from build123d import *

# Parameters (mm, degrees)
SKETCH_1_R           = 155
EXTRUDE_1_DEPTH      = 5
SKETCH_16_R          = 1.5
CUT_EXTRUDE_15_DEPTH = 220.260119493
SKETCH_17_R          = 1.5
SKETCH_17_R_2        = 20.5
CUT_EXTRUDE_16_DEPTH = 220.260119493
SKETCH_19_R          = 2
SKETCH_19_R_2        = 1.5
CUT_EXTRUDE_17_DEPTH = 220.260119493
CUT_EXTRUDE_18_DEPTH = 220.260119493
SKETCH_21_R          = 1.5
CUT_EXTRUDE_19_DEPTH = 220.260119493
SKETCH_22_R          = 1.5
SKETCH_22_W          = 78
SKETCH_22_H          = 51
CUT_EXTRUDE_20_DEPTH = 220.260119493


with BuildPart() as part:
    # 草图1 → 凸台-拉伸1 (new body)
    with BuildSketch(Plane.XY):
        Circle(SKETCH_1_R)
    extrude(amount=EXTRUDE_1_DEPTH)

    # 草图16 → 切除-拉伸15 (cut, through all)
    with BuildSketch(Plane.XY.offset(5)):
        with Locations((0, 148)):
            Circle(SKETCH_16_R)
        with Locations((104.651803616, 104.651803616)):
            Circle(SKETCH_16_R)
        with Locations((148, 0)):
            Circle(SKETCH_16_R)
        with Locations((104.651803616, -104.651803616)):
            Circle(SKETCH_16_R)
        with Locations((0, -148)):
            Circle(SKETCH_16_R)
        with Locations((-104.651803616, -104.651803616)):
            Circle(SKETCH_16_R)
        with Locations((-148, 0)):
            Circle(SKETCH_16_R)
        with Locations((-104.651803616, 104.651803616)):
            Circle(SKETCH_16_R)
    extrude(amount=-CUT_EXTRUDE_15_DEPTH, mode=Mode.SUBTRACT)

    # 草图17 → 切除-拉伸16 (cut, through all)
    with BuildSketch(Plane.XY.offset(5)):
        with Locations((-80, -75)):
            Circle(SKETCH_17_R)
        with Locations((-80, -125)):
            Circle(SKETCH_17_R)
        with Locations((-80, -100)):
            Circle(SKETCH_17_R_2)
    extrude(amount=-CUT_EXTRUDE_16_DEPTH, mode=Mode.SUBTRACT)

    # 草图19 → 切除-拉伸17 (cut, through all)
    with BuildSketch(Plane.XY.offset(5)):
        with Locations((51.7, -68.3)):
            Circle(SKETCH_19_R)
        with Locations((43.2, -120.3)):
            Circle(SKETCH_19_R)
        with Locations((-43.2, -120.3)):
            Circle(SKETCH_19_R)
        with Locations((-51.7, -68.3)):
            Circle(SKETCH_19_R)
        with Locations((25.1, -72.7)):
            Circle(SKETCH_19_R_2)
        with Locations(Location((25.1, -122.7, 0), (0, 0, 180))):
            Circle(SKETCH_19_R_2)
        with Locations((-24.9, -122.7)):
            Circle(SKETCH_19_R_2)
        with Locations(Location((-24.9, -72.7, 0), (0, 0, 180))):
            Circle(SKETCH_19_R_2)
    extrude(amount=-CUT_EXTRUDE_17_DEPTH, mode=Mode.SUBTRACT)

    # 草图20 → 切除-拉伸18 (cut, through all)
    with BuildSketch(Plane.XY.offset(5)):
        with BuildLine():
            Line((-75, 42), (75, 42))
            ThreePointArc((75, 42), (82.071067812, 39.071067812), (85, 32))
            Line((85, 32), (85, -50))
            ThreePointArc((85, -50), (82.071067812, -57.071067812), (75, -60))
            Line((75, -60), (-75, -60))
            ThreePointArc((-75, -60), (-82.071067812, -57.071067812), (-85, -50))
            Line((-85, -50), (-85, 32))
            ThreePointArc((-85, 32), (-82.071067812, 39.071067812), (-75, 42))
        make_face()
    extrude(amount=-CUT_EXTRUDE_18_DEPTH, mode=Mode.SUBTRACT)

    # 草图21 → 切除-拉伸19 (cut, through all)
    with BuildSketch(Plane.XY.offset(5)):
        with Locations((95, 16)):
            Circle(SKETCH_21_R)
        with Locations((120, 16)):
            Circle(SKETCH_21_R)
        with Locations(Location((120, -34, 0), (0, 0, 180))):
            Circle(SKETCH_21_R)
        with Locations(Location((95, -34, 0), (0, 0, 180))):
            Circle(SKETCH_21_R)
        with Locations((-120, -34)):
            Circle(SKETCH_21_R)
        with Locations((-95, -34)):
            Circle(SKETCH_21_R)
        with Locations(Location((-120, 16, 0), (0, 0, 180))):
            Circle(SKETCH_21_R)
        with Locations(Location((-95, 16, 0), (0, 0, 180))):
            Circle(SKETCH_21_R)
    extrude(amount=-CUT_EXTRUDE_19_DEPTH, mode=Mode.SUBTRACT)

    # 草图22 → 切除-拉伸20 (cut, through all)
    with BuildSketch(Plane.XY.offset(5)):
        with Locations((-44, 129.5)):
            Circle(SKETCH_22_R)
        with Locations((44, 129.5)):
            Circle(SKETCH_22_R)
        with Locations((44, 70.5)):
            Circle(SKETCH_22_R)
        with Locations((-44, 70.5)):
            Circle(SKETCH_22_R)
        with Locations((0, 100)):
            Rectangle(SKETCH_22_W, SKETCH_22_H)
    extrude(amount=-CUT_EXTRUDE_20_DEPTH, mode=Mode.SUBTRACT)


solid = part.part
Build history of the part. All positions in model axes, mm. A direction names the side the tool comes from. Coordinates: 2 decimals unless noted, no trailing zeros. Order: outer loops, then holes, each group sorted by start corner. A loop starts at its lowest first (then second) coordinate and runs counter-clockwise, first axis right, second up. Notation, with made-up numbers: M 30.25,89 L 64.25,89 A15 cw 64.25,109 Z; hole C -20,58 d3. An arc over 180 degrees is marked long. One line per question, with ' | ' between items. Start each with the question number.
Q1. Saw through at D-D (y = 49). List the corners of the cut face in (x, z), then the cut area to 3 significant figures.
Q2. 3-axis set-ups, long thin cutter, end or side, ignore diameter. For faces 1 (the face through (-2, -67, 5)), 2 (the face through (-81.99, -57.15, 2.54)): which of +Z, -Z, +X, -X, +Y, -Y reach the whole face in a straight line?
Q3. Two-plate mould, pull along Y, no slides. Class faces 3 (the face through (-2, -67, 0)), 4 (the face through (81.99, 39.15, 2.54)), 5 (the face through (-33.601, -151.314, 2.465)): +Y half, -Y half, draft (parallel to the pull), parting line (faces both ways), or undercut.
Q4. Flat gauge pins, fed straight in: pin 1 Ø2.5 at (x, z) = (30, 2) entering from +Y; pin 2 Ø2 at (y, z) = (-39.5, 3) entering from -X; pin 3 Ø2.5 at (x, z) = (-27, 3.5) entering from -Y; pin 4 Ø2.5 at (x, y) = (-80, -75) entering from -Z. Where does each tip first touch, or does it go through?
Q5. Saw through at C-C (z = 1.8). Count the separate pieces of the cut face and the enclosed holes in it, then the cut area to 3 significant figures.
Q6. Saw through at B-B (y = 112). List the corners of the cut face in (x, z).
Q7. Saw through at A-A (y = -10.5). List the corners of the cut face in (x, z), then the cut area to 3 significant figures.
Q8. Probe L1, parallel to Y at x = 0, z = 1.2; L2, parallel to X at y = 128.5, z = 2.25; L3, parallel to X at y = 129.5, z = 1.95. List the from-to ranges inside material, lowest first. Write a range as from..to.
Check values:
1) outline: M -147.05,0 L 147.05,0 L 147.05,5 L -147.05,5 Z | area: 1,470 mm2
2) face 1: +Z, +X, -X, +Y, -Y | face 2: +Z, -Z
3) face 3: draft | face 4: undercut | face 5: parting line
4) pin 1: stops at y = 152.31 | pin 2: stops at x = -150.14 | pin 3: stops at y = -152.85 | pin 4: passes through
5) separate pieces: 1 | enclosed holes: 33 | area: 52,700 mm2
6) outline: M -107.15,0 L -39,0 L -39,5 L -107.15,5 Z; M 39,0 L 107.15,0 L 107.15,5 L 39,5 Z
7) outline: M -154.64,0 L -85,0 L -85,5 L -154.64,5 Z; M 85,0 L 154.64,0 L 154.64,5 L 85,5 Z | area: 696 mm2
8) L1: y = -155..-149.5, -146.5..-60, 42..74.5, 125.5..146.5, 149.5..155 | L2: x = -86.68..-45.12, -42.88..42.88, 45.12..86.68 | L3: x = -85.17..-45.5, -42.5..42.5, 45.5..85.17
